Verification items for the finished model (mm, model axes). Round coordinates to 2 decimals unless told otherwise and drop trailing zeros. Order: outer loops, then holes, each group sorted by start corner. A loop starts at its lowest first (then second) coordinate and runs counter-clockwise, first axis right, second up. Notation, with made-up numbers: M 69.25,64 L 124.25,64 A34 ccw 124.25,95 Z; hole C 23.25,56 d7. An arc over 180 degrees is marked long. Use CSV: the item, a comma, the result in double quotes. Start each with the question number.
Q1. Gauge pin test, flat ends, axial feed: pin 1 Ø6 at (y, z) = (-8, 2.5) entering from -X; pin 2 Ø1 at (x, z) = (2.5, 8.5) entering from -Y; pin 3 Ø12 at (x, y) = (-5.5, 0) entering from -Z. Record the tip position at first contact, or that the pin passes through.
Q2. Sectioned sample at A-A (x = 0). Enter the section's corners in (y, z).
Q3. Scan lines: line 1 (X direction, y = 0.75, z = 5.5); line 2 (X direction, y = 0.5, z = 1.25); line 3 (Y direction, x = 5.5, z = 2). Record each from-to range of solid material in increasing order.
Q4. Mould release check, pull along Z, two halves, no side actions. Record for faces 1 (the face through (0, 0, 0)), 2 (the face through (-2.93, 13.18, 1.48)), 3 (the face through (12.104, -5.019, 6.898)), 4 (the face through (0, 0, 10)): +Z half, -Z half, draft (parallel to the pull), parting line (faces both ways), or undercut.
Q5. Sectioned sample at B-B (z = 1.25). Enter the section's corners in (x, y).
```python
from build123d import *

# Parameters (mm, degrees)
F0_R     = 12.5
F1_DEPTH = 10
F1_TAPER = -5
F2_R     = 13.5
F3_DEPTH = 3


# Not quite as in the source:
# - a fillet or chamfer that OpenCascade refuses, or shapes differently, is made with other operations: its cross-section is extruded or revolved along the edge and cut away or added


with BuildPart() as f1:
    # F0 (on Top) → F1 (new body)
    with BuildSketch(Plane.XY):
        Circle(F0_R)
    extrude(amount=F1_DEPTH, taper=F1_TAPER)

    # F2 (on face) → F3 (join)
    with BuildSketch(Plane(origin=(0, 0, 0), x_dir=(1, 0, 0), z_dir=(0, 0, -1))):
        Circle(F2_R)
    extrude(amount=-F3_DEPTH)

    # F4: fillet of radius 5 on 1 edges, made by hand

    # F4_s1 → F4_t2 (revolve)
    with BuildSketch(Plane.XZ):
        with BuildLine():
            ThreePointArc((13.5, 3), (13.0638190953, 4.2967665116), (12.9954672306, 5.6632163606))
            Line((12.9954672306, 5.6632163606), (12.8958477608, 5.6719319348))
            Line((12.8958477608, 5.6719319348), (12.6628465208, 3.0087155743))
            Line((12.6628465208, 3.0087155743), (12.7624659906, 2.9))
            ThreePointArc((12.7624659906, 2.9), (13.1312329953, 2.9), (13.4104711856, 2.9554512471))
            Line((13.4104711856, 2.9554512471), (13.5, 3))
        make_face()
    revolve(axis=Axis((0, 0, 3), (0, 0, 1)))


solid = f1.part
```
Verdict:
1,pin 1,"stops at x = -12.54"
1,pin 2,"stops at y = -13.1"
1,pin 3,"stops at z = 0"
2,outline,"M -13.5,0 L 13.5,0 L 13.5,3 A5 cw 13,5.66 L 13.37,10 L -13.37,10 L -13,5.66 A5 cw -13.5,3 Z"
3,line 1,"x = -12.96 to 12.96"
3,line 2,"x = -13.49 to 13.49"
3,line 3,"y = -12.33 to 12.33"
4,face 1,"-Z half"
4,face 2,"draft"
4,face 3,"undercut"
4,face 4,"+Z half"
5,outline,"C 0,0 d27"
